CAD build for the part. Positions are in the model's coordinates, mm. A direction names the side the tool comes from. Round coordinates to 2 decimals unless told otherwise and drop trailing zeros. Write each loop counter-clockwise with the first axis right and the second up, starting at its lowest first coordinate (ties: lowest second). Pieces come first, ordered by that corner, then holes. Notation, with made-up numbers: (82, -36) -> (134, -36) arc R22 cw to (134, -25) -> close; hole circle Ø2 at (36.25, -21.5). An arc over 180 degrees is marked (long way). Put each result on its own line as item: value. Start each with the question number.
1. Saw through at B-B on y = -5.5. List the corners of the cut face in (x, z), and give its area (3 significant figures).
2. Flat gauge pins, fed straight in: P1, Ø4, axis at x = 3.5, y = -7.5, coming from the -Z side; P2, Ø5, axis at y = -1, z = -3.5, coming from the +X side; P3, Ø2, axis at x = -2, z = 2, coming from the +Y side; P4, Ø0.7, axis at x = 0.5, z = 2, coming from the -Y side. Where does each tip first touch, or does it go through?
3. 3-axis set-ups, long thin cutter, end or side, ignore diameter. For faces 4 (the flat face through (3.16, -5.67, 1.15)), 5 (the flat face through (1, -7.6, 3)), 6 (the conical face through (1.301, -5.268, -2.306)), 7 (the flat face through (-2.56, -5.67, -2.15)): which of +Z, -Z, +X, -X, +Y, -Y reach the whole face in a straight line?
4. Saw through at C-C on y = -6.5. List the corners of the cut face in (x, z).
5. Saw through at A-A on z = 0. List the corners of the cut face in (x, y).
6. Saw through at D-D on y = -1.75. List the corners of the cut face in (x, z), and give its area (3 significant figures).
7. Drill centre lines: line 1 (Z direction, x = 3.25, y = -3.5); line 2 (X direction, y = -4.75, z = -2); line 3 (Z direction, x = 2.5, y = -5). Where is each one in solid material? Low to high. Write a range as from..to.
8. Pull direction Z, two halves, no side cores. Call faces 1 (the conical face through (1.637, -9.135, 2.773)), 2 (the cylindrical face through (4.783, -1.521, -1.062)), 3 (the cylindrical face through (1.917, -6.549, -3.396)): pulls with the +Z half, pulls with the -Z half, needs draft (parallel to the pull), parting line crosses it, or undercut.
from build123d import *

# Parameters (mm, degrees)
F3_DEPTH = 10


with BuildPart() as f1:
    # F0 (on Right) → F1 (revolve)
    with BuildSketch(Plane.YZ):
        Polygon((-7.6, 2.8), (-3, 2.5), (0, 4.4), (0, 4.9), (-3, 4.9), (-3, 3.9), (-10, 3.9), (-8.6, 2.8), (-8.6, 3.4), (-7.6, 3.4), align=None)
    revolve(axis=Axis((0, -6.9740121253, 0), (0, -1, 0)))

    # F2 (on face) → F3 (cut)
    with BuildSketch(Plane.XZ.offset(3)):
        with BuildLine():
            Line((-2.9875733282, 2.5068716778), (0, 0))
            Line((0, 0), (-0.6772278929, 3.8407502367))
            ThreePointArc((-0.6772278929, 3.8407502367), (-1.95, 3.3774990748), (-2.9875733282, 2.5068716778))
        make_face()
        with BuildLine():
            Line((3.6648012211, 1.333878559), (0, 0))
            Line((0, 0), (3.9, 0))
            ThreePointArc((3.9, 0), (3.8407502367, 0.6772278929), (3.6648012211, 1.333878559))
        make_face()
        with BuildLine():
            Line((3.9, 0), (0, 0))
            Line((0, 0), (3.6648012211, -1.333878559))
            ThreePointArc((3.6648012211, -1.333878559), (3.8407502367, -0.6772278929), (3.9, 0))
        make_face()
        with BuildLine():
            Line((-0.6772278929, -3.8407502367), (0, 0))
            Line((0, 0), (-2.9875733282, -2.5068716778))
            ThreePointArc((-2.9875733282, -2.5068716778), (-1.95, -3.3774990748), (-0.6772278929, -3.8407502367))
        make_face()
        with BuildLine():
            Line((-0.8508760706, 4.8255579898), (-0.6772278929, 3.8407502367))
            ThreePointArc((-0.6772278929, 3.8407502367), (1.95, 3.3774990748), (3.6648012211, 1.333878559))
            Line((3.6648012211, 1.333878559), (4.6044938419, 1.6758987023))
            ThreePointArc((4.6044938419, 1.6758987023), (2.45, 4.2435244785), (-0.8508760706, 4.8255579898))
        make_face()
        with BuildLine():
            ThreePointArc((3.6648012211, 1.333878559), (3.8407502367, 0.6772278929), (3.9, 0))
            Line((3.9, 0), (4.9, 0))
            ThreePointArc((4.9, 0), (4.8255579898, 0.8508760706), (4.6044938419, 1.6758987023))
            Line((4.6044938419, 1.6758987023), (3.6648012211, 1.333878559))
        make_face()
        with BuildLine():
            Line((4.9, 0), (3.9, 0))
            ThreePointArc((3.9, 0), (3.8407502367, -0.6772278929), (3.6648012211, -1.333878559))
            Line((3.6648012211, -1.333878559), (4.6044938419, -1.6758987023))
            ThreePointArc((4.6044938419, -1.6758987023), (4.8255579898, -0.8508760706), (4.9, 0))
        make_face()
        with BuildLine():
            ThreePointArc((3.6648012211, -1.333878559), (1.95, -3.3774990748), (-0.6772278929, -3.8407502367))
            Line((-0.6772278929, -3.8407502367), (-0.8508760706, -4.8255579898))
            ThreePointArc((-0.8508760706, -4.8255579898), (2.45, -4.2435244785), (4.6044938419, -1.6758987023))
            Line((4.6044938419, -1.6758987023), (3.6648012211, -1.333878559))
        make_face()
    extrude(amount=F3_DEPTH, mode=Mode.SUBTRACT)


solid = f1.part
Return value:
1. outline: (-2.99, -2.51) -> (-2.04, -1.71) arc R2.66 cw to (-2.04, 1.71) -> (-2.99, 2.51) arc R3.9 ccw to start; (-0.68, -3.84) arc R3.9 ccw to (3.66, -1.33) -> (2.5, -0.91) arc R2.66 cw to (-0.46, -2.62) -> close; (-0.68, 3.84) -> (-0.46, 2.62) arc R2.66 cw to (2.5, 0.91) -> (3.66, 1.33) arc R3.9 ccw to start
1. area: 17.0 mm^2
2. P1: stops at z = -3.6
2. P2: stops at x = 4.8
2. P3: stops at y = -0.9
2. P4: passes through
3. face 4: +X, -Y
3. face 5: none
3. face 6: -Y
3. face 7: -Z, -Y
4. outline: (-2.99, -2.51) -> (-2.09, -1.75) arc R2.73 cw to (-2.09, 1.75) -> (-2.99, 2.51) arc R3.9 ccw to start; (-0.68, -3.84) arc R3.9 ccw to (3.66, -1.33) -> (2.56, -0.93) arc R2.73 cw to (-0.47, -2.69) -> close; (-0.68, 3.84) -> (-0.47, 2.69) arc R2.73 cw to (2.56, 0.93) -> (3.66, 1.33) arc R3.9 ccw to start
5. outline: (-4.9, -3) -> (-3.9, -3) -> (-3.9, -10) -> (-2.8, -8.6) -> (-3.4, -8.6) -> (-3.4, -7.6) -> (-2.8, -7.6) -> (-2.5, -3) -> (-4.4, 0) -> (-4.9, 0) -> close; (2.5, -3) -> (4.9, -3) -> (4.9, 0) -> (4.4, 0) -> close
6. outline: circle Ø9.8 at (0, 0); hole circle Ø6.58 at (0, 0)
6. area: 41.4 mm^2
7. line 1: z = -2.16..-1.18, 1.18..2.16
7. line 2: x = -3.35..-2.38, 1.68..3.35
7. line 3: z = -2.99..-0.91, 0.91..2.99
8. face 1: undercut
8. face 2: parting line crosses it
8. face 3: pulls with the -Z half
